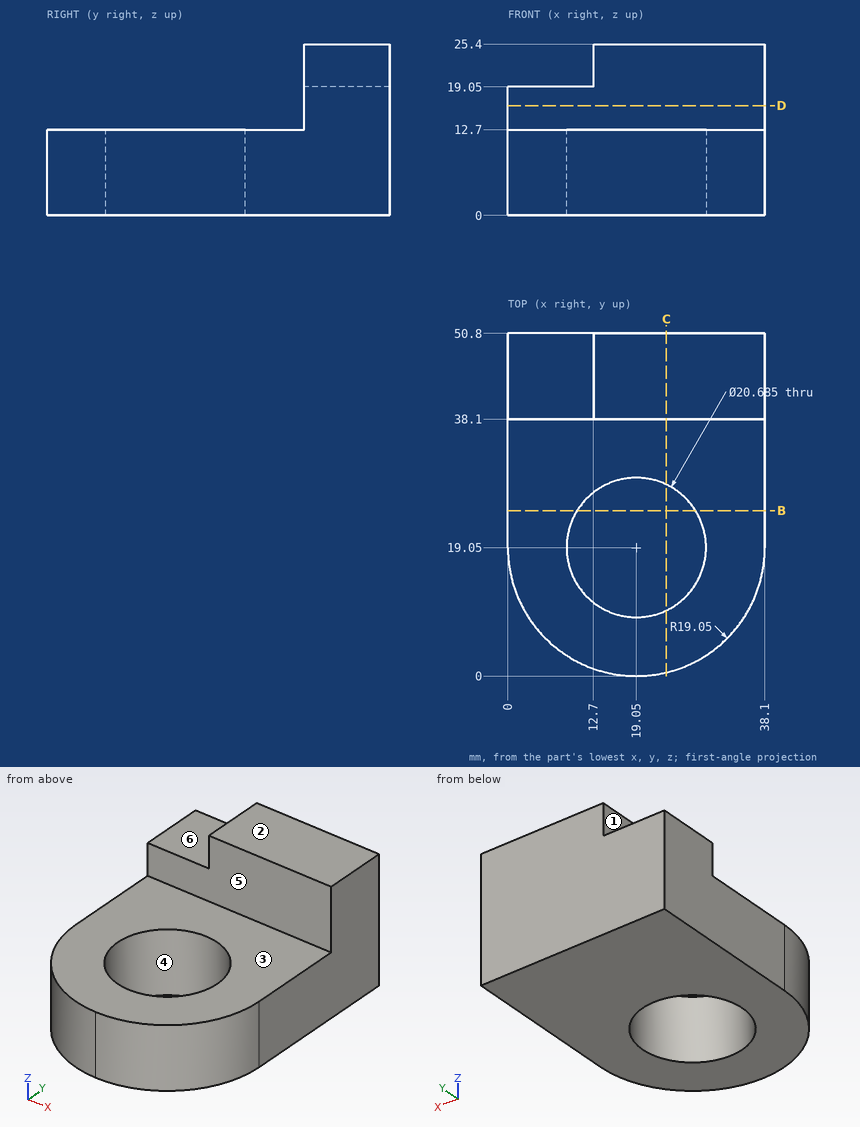
Design review of the part shown in the three views and the two pictorial views. Dimensions are in mm from the part's minimum x, y and z. A direction names the side the tool comes from. Give positions to 0.01 mm unless a question says otherwise; leave off trailing zeros. Write each loop counter-clockwise with the first axis right and the second up, starting at its lowest first coordinate (ties: lowest second). Pieces come first, ordered by that corner, then holes. Notation, with made-up numbers: (79, 39) - (91, 39) arc R24 cw to (91, 54) - close; hole circle Ø10 at (64.5, 36). An arc over 180 degrees is marked (long way). Return JSON: item names as keys, results as strings. Group by question number.
(1) Machinability: for the marked faces 1, 2 and 3, which of the approach directions +Z, -Z, +X, -X, +Y, -Y give a long, thin tool a straight path to every point of the face, cutting with its end or side? Answer none if there is none.
(2) We need section C-C, the plane x = 23.5. Give the boundary of the cut face in (y, z).
(3) Mouldability with a two-part tool opening along Y and no side actions: class the marked faces 4, 5 and 6 as +Y half, -Y half, draft (parallel to the pull), parting line (faces both ways), or undercut.
(4) Insertion check: pin 1 (4 mm diameter, centred on x = 7, y = 42, fed in from +Z); pin 2 (3 mm diameter, centred on y = 45.5, z = 23, fed in from -X); pin 3 (2 mm diameter, centred on x = 15.5, y = 27.5, fed in from -Z); pin 4 (6.5 mm diameter, centred on x = 12.5, z = 21.5, fed in from -Y). Each pin has a flat end and moves straight along its axis. Give the tip position at first contact, or say it passes through.
(5) We need section D-D, the plane z = 16.25. Give the boundary of the cut face in (x, y), then the cut area to 3 significant figures.
(6) To check wall thickness, follow probe 1 along Z at (x, y) = (8, 48); probe 2 along Z at (x, y) = (12, 31); probe 3 along Y at (x, z) = (34.5, 20.25). State the ranges of each line that lie inside material, in increasing order.
(7) We need section B-B, the plane y = 24.5. Give the boundary of the cut face in (x, z).
Reported:
{
 "1": {"face 1": "+Z, -X, +Y, -Y", "face 2": "+Z, +X, -X, +Y, -Y", "face 3": "+Z, +X, -X, -Y"},
 "2": {"outline": "(0.53, 0) - (9.71, 0) - (9.71, 12.7) - (0.53, 12.7) - close; (28.39, 0) - (50.8, 0) - (50.8, 25.4) - (38.1, 25.4) - (38.1, 12.7) - (28.39, 12.7) - close"},
 "3": {"face 4": "undercut", "face 5": "-Y half", "face 6": "draft"},
 "4": {"pin 1": "stops at z = 19.05", "pin 2": "stops at x = 12.7", "pin 3": "passes through", "pin 4": "stops at y = 38.1"},
 "5": {"outline": "(0, 38.1) - (38.1, 38.1) - (38.1, 50.8) - (0, 50.8) - close", "area": "484 mm2"},
 "6": {"probe 1": "z = 0 to 19.05", "probe 2": "z = 0 to 12.7", "probe 3": "y = 38.1 to 50.8"},
 "7": {"outline": "(0, 0) - (10.26, 0) - (10.26, 12.7) - (0, 12.7) - close; (27.84, 0) - (38.1, 0) - (38.1, 12.7) - (27.84, 12.7) - close"}
}
